```python
from build123d import *

# Parameters (mm, degrees)
SKETCH1_W             = 92
SKETCH1_H             = 92
SKETCH1_R             = 44.3
SKETCH1_R_2           = 2.25
BOSS_EXTRUDE1_DEPTH   = 12.65
SKETCH1_R_3           = 18.5
BOSS_EXTRUDE1_2_DEPTH = 12.65
BOSS_EXTRUDE2_START   = -3
BOSS_EXTRUDE2_DEPTH   = 3
CIRPATTERN1_COUNT     = 4


with BuildPart() as part:
    # Sketch1 → Boss-Extrude1 (new, symmetric)
    with BuildSketch(Plane.XY):
        Rectangle(SKETCH1_W, SKETCH1_H)
        Circle(SKETCH1_R, mode=Mode.SUBTRACT)
        with Locations((-41.188970004, -41.188970004)):
            Circle(SKETCH1_R_2, mode=Mode.SUBTRACT)
        with Locations((41.188970004, -41.188970004)):
            Circle(SKETCH1_R_2, mode=Mode.SUBTRACT)
        with Locations((41.188970004, 41.188970004)):
            Circle(SKETCH1_R_2, mode=Mode.SUBTRACT)
        with Locations((-41.188970004, 41.188970004)):
            Circle(SKETCH1_R_2, mode=Mode.SUBTRACT)
    extrude(amount=BOSS_EXTRUDE1_DEPTH, both=True)



with BuildPart() as body_2:
    # Sketch1 → Boss-Extrude1 2 (new, symmetric)
    with BuildSketch(Plane.XY):
        Circle(SKETCH1_R_3)
    extrude(amount=BOSS_EXTRUDE1_2_DEPTH, both=True)


with BuildPart() as part_1:
    add(part.part)

    add(body_2.part)  # Boss-Extrude2 merges body 2
    # Sketch2 → Boss-Extrude2 (add)
    with BuildSketch(Plane.XY.offset(12.65).offset(BOSS_EXTRUDE2_START)):
        with BuildLine():
            Line((0, 18.5), (20.677955159, 39.177955159))
            ThreePointArc((20.677955159, 39.177955159), (22.482427755, 38.171068131), (24.237983576, 37.081129327))
            Line((24.237983576, 37.081129327), (4.975286421, 17.818432171))
            ThreePointArc((4.975286421, 17.818432171), (2.510876823, 18.328816044), (0, 18.5))
        make_face()
    boss_extrude2 = extrude(amount=BOSS_EXTRUDE2_DEPTH)

    # CirPattern1: Boss-Extrude2 ×4 about axis
    cirpattern1_axis = Axis((0, 0, 0), (0, 0, 1))
    for i in range(1, CIRPATTERN1_COUNT):
        add(boss_extrude2.rotate(cirpattern1_axis, i * 360 / CIRPATTERN1_COUNT))


solid = part_1.part
```
The model under review builds one solid part; all positions refer to its coordinate system, in mm. A direction names the side the tool comes from. Coordinates: 2 decimals unless noted, no trailing zeros. Write each loop counter-clockwise with the first axis right and the second up, starting at its lowest first coordinate (ties: lowest second). Pieces come first, ordered by that corner, then holes.
1) We need section B-B on z = 3.5. State the section outline as (x, y) points.
2) We need section A-A on y = -31. State the section outline as (x, z) points, then the cut area to 3 significant figures.
3) Machinability: for faces 1 (the face through (12, 28, 9.65)), 2 (the face through (46, -1, 0)), 3 (the face through (-27.585, 14.741, 11.129)), which of the approach directions +Z, -Z, +X, -X, +Y, -Y give a long, thin tool a straight path to every point of the face, cutting with its end or side? Answer none if there is none.
4) We need section C-C on x = 27. State the section outline as (y, z) points, then the cut area to 3 significant figures.
5) Clearance check with flat-ended pins moving along their axes: pin 1 Ø3.5 at (x, y) = (41.19, -41.19) entering from -Z; pin 2 Ø17 at (x, y) = (8.5, 26) entering from -Z. State where each tip first meets the part, or that it passes through.
6) The part is to be moulded in two halves that separate along X. For faces 4 (the face through (-46, -1, 0)), 5 (the face through (-1, -46, 0)), 6 (the face through (42.227, 39.193, -0.177)), say which applies: pulls with the +X half, pulls with the -X half, needs draft (parallel to the pull), parting line crosses it, or undercut.
7) To check wall thickness, follow probe 1 along Y at (x, z) = (0, -6.5); probe 2 along X at (y, z) = (0.5, 3.5); probe 3 along Y at (x, z) = (8, -10.25). State the ranges of each line that lie inside material, in increasing order.
8) We need section D-D on y = -15.5. State the section outline as (x, z) points, then the cut area to 3 significant figures.
Answer list:
1. outline: (-46, -46) - (46, -46) - (46, 46) - (-46, 46) - close; circle Ø37 at (0, 0); hole circle Ø88.6 at (0, 0); hole circle Ø4.5 at (-41.19, -41.19); hole circle Ø4.5 at (-41.19, 41.19); hole circle Ø4.5 at (41.19, -41.19); hole circle Ø4.5 at (41.19, 41.19)
2. outline: (-46, -12.65) - (-31.65, -12.65) - (-31.65, 12.65) - (-46, 12.65) - close; (-18.16, 9.65) - (-12.5, 9.65) - (-12.5, 12.65) - (-18.16, 12.65) - close; (31.65, -12.65) - (46, -12.65) - (46, 12.65) - (31.65, 12.65) - close
2. area: 743 mm2
3. face 1: -Z
3. face 2: +Z, -Z, +X, +Y, -Y
3. face 3: +Z, -Z
4. outline: (-46, -12.65) - (-35.12, -12.65) - (-35.12, 12.65) - (-46, 12.65) - close; (-14.16, 9.65) - (-8.5, 9.65) - (-8.5, 12.65) - (-14.16, 12.65) - close; (35.12, -12.65) - (46, -12.65) - (46, 12.65) - (35.12, 12.65) - close
4. area: 567 mm2
5. pin 1: passes through
5. pin 2: stops at z = 9.65
6. face 4: pulls with the -X half
6. face 5: needs draft
6. face 6: undercut
7. probe 1: y = -46 to -44.3, -18.5 to 18.5, 44.3 to 46
7. probe 2: x = -46 to -44.3, -18.49 to 18.49, 44.3 to 46
7. probe 3: y = -46 to -43.57, -16.68 to 16.68, 43.57 to 46
8. outline: (-46, -12.65) - (-41.5, -12.65) - (-41.5, 12.65) - (-46, 12.65) - close; (-10.1, -12.65) - (10.1, -12.65) - (10.1, 12.65) - (-10.1, 12.65) - close; (28.34, 9.65) - (34, 9.65) - (34, 12.65) - (28.34, 12.65) - close; (41.5, -12.65) - (46, -12.65) - (46, 12.65) - (41.5, 12.65) - close
8. area: 756 mm2
